Can you work these out from the model? Positions are in its coordinate system, mm. A direction names the side the tool comes from. Give positions to 0.01 mm unless a question says otherwise; leave off trailing zeros. Loops run counter-clockwise (first coordinate to the right, second up) from the corner with the lowest first, then second, coordinate; pieces in that order, holes last. Notation, with made-up numbers: M -22.5,-15.75 L 8.5,-15.75 A14 ccw 8.5,3.25 Z; hole C 46,-10.75 d3. An arc over 180 degrees is marked long. Put each result on its own line as item: value. Start each with the question number.
1) Imagine slicing it at A-A (x = 6). Write out the boundary of the cut face in (y, z), then the cut area to 3 significant figures.
2) Imagine slicing it at B-B (y = -6). State how many separate pieces and enclosed holes the cut face has, then the cut area to 3 significant figures.
3) For faces 1 (the cylindrical face through (15.32, -11.43, 4.4)), 2 (the cylindrical face through (1.5, -1.43, 2.49)), 3 (the cylindrical face through (15.32, -11.43, 0.6)), 4 (the cylindrical face through (72.18, -15.99, 4.43)), 5 (the cylindrical face through (1.43, -10.5, 2.49)), which set-ups out of +Z, -Z, +X, -X, +Y, -Y let a thin tool reach every point of the face, with its end or its side?
4) Please list where these lines run through material, in increasing order: line 1 along Y through (x, z) = (14, 1.85); line 2 along Y through (x, z) = (22.5, 4.65); line 3 along Y through (x, z) = (10, 0.9). Write a range as from..to.
5) For P1, Ø1, axis at x = 60.5, z = 3, coming from the +Y side; P2, Ø4.5, axis at x = 22, y = -6, coming from the +Z side; P3, Ø5, axis at x = 6, y = -6, coming from the -Z side, each with a flat end and sliding along its axis, tell me the tip position at first contact or that it passes through.
6) If we mould it in two halves opening along X, with no side actions, what happens to faces 6 (the cylindrical face through (81.685, -21.377, 4.43)), 7 (the cylindrical face through (0.57, -5.99, 0.6)), 8 (the cylindrical face through (12.4, -7.2, 2.5))? For each: +X half, -X half, draft (parallel to the pull), parting line (faces both ways), or undercut.
from build123d import *

# Parameters (mm, degrees)
F0_W         = 25
F0_H         = 12
F0_W_2       = 15
F1_DEPTH     = 5
F2_R         = 2
F3_DEPTH     = 5.001
F4_R         = 2
F5_T1_DEPTH  = 5
F5_T4_ANGLE  = 90
F5_T6_ANGLE  = 90
F5_T8_ANGLE  = 90
F5_T10_ANGLE = 90
F5_T12_ANGLE = 90
F5_T14_ANGLE = 90
F5_T16_ANGLE = 90
F5_T18_ANGLE = 90
F6_SIZE      = 1


# Not quite as in the source:
# - a fillet or chamfer that OpenCascade refuses, or shapes differently, is made with other operations: its cross-section is extruded or revolved along the edge and cut away or added


with BuildPart() as f1:
    # F0 (on Top) → F1 (new body)
    with BuildSketch(Plane.XY):
        with Locations((12.5, -6)):
            Rectangle(F0_W, F0_H)
        Polygon((67.2861679354, -15.3909064497), (25, 0), (25, -12), (67.2861679354, -27.3909064497), align=None)
        with Locations((74.7861679354, -21.3909064497)):
            Rectangle(F0_W_2, F0_H)
    extrude(amount=F1_DEPTH)

    # F2 (on face) → F3 (cut, through all)
    with BuildSketch(Plane.XY.offset(5)):
        with Locations((6, -6)):
            Circle(F2_R)
        with Locations((76.2861679354, -21.3909064497)):
            Circle(F2_R)
        with Locations((14, -6)):
            Circle(F2_R)
        with Locations((22, -6)):
            Circle(F2_R)
        with Locations((68.2861679354, -21.3909064497)):
            Circle(F2_R)
    extrude(amount=-F3_DEPTH, mode=Mode.SUBTRACT)

    # F4
    f4_edges = [f1.edges().sort_by_distance(p)[0] for p in [
        (46.143084, -7.695453, 5),
        (74.786168, -15.390906, 5),
        (82.286168, -21.390906, 5),
        (74.786168, -27.390906, 5),
        (46.143084, -19.695453, 5),
        (12.5, -12, 5),
        (0, -6, 5),
        (12.5, 0, 5),
        (12.5, -12, 0),
        (0, -6, 0),
        (12.5, 0, 0),
        (46.143084, -7.695453, 0),
        (46.143084, -19.695453, 0),
        (74.786168, -27.390906, 0),
        (74.786168, -15.390906, 0),
        (82.286168, -21.390906, 0),
    ]]
    fillet(f4_edges, radius=F4_R)

    # F5: fillet of radius 5 on 4 edges, made by hand

    # F5_s2 → F5_t1 (cut)
    with BuildSketch(Plane.XY):
        with BuildLine():
            ThreePointArc((77.2861679354, -15.3909064497), (80.8217018413, -16.8553725437), (82.2861679354, -20.3909064497))
            Line((82.2861679354, -20.3909064497), (82.2861679354, -15.3909064497))
            Line((82.2861679354, -15.3909064497), (77.2861679354, -15.3909064497))
        make_face()
        with BuildLine():
            ThreePointArc((82.2861679354, -22.3909064497), (80.8217018413, -25.9264403556), (77.2861679354, -27.3909064497))
            Line((77.2861679354, -27.3909064497), (82.2861679354, -27.3909064497))
            Line((82.2861679354, -27.3909064497), (82.2861679354, -22.3909064497))
        make_face()
        with BuildLine():
            ThreePointArc((0, -7), (1.4644660941, -10.5355339059), (5, -12))
            Line((5, -12), (0, -12))
            Line((0, -12), (0, -7))
        make_face()
        with BuildLine():
            ThreePointArc((5, 0), (1.4644660941, -1.4644660941), (0, -5))
            Line((0, -5), (0, 0))
            Line((0, 0), (5, 0))
        make_face()
    extrude(amount=F5_T1_DEPTH, mode=Mode.SUBTRACT)

    # F5_s3 → F5_t4 (revolve, cut)
    with BuildSketch(Plane.XZ.offset(5)):
        with BuildLine():
            ThreePointArc((2, 0), (0.5857864376, 0.5857864376), (0, 2))
            Line((0, 2), (0, 0))
            Line((0, 0), (2, 0))
        make_face()
    revolve(axis=Axis((5, -5, 0), (0, 0, -1)), revolution_arc=F5_T4_ANGLE, mode=Mode.SUBTRACT)

    # F5_s5 → F5_t6 (revolve, cut)
    with BuildSketch(Plane.YZ.offset(5)):
        with BuildLine():
            ThreePointArc((-10, 0), (-11.4142135624, 0.5857864376), (-12, 2))
            Line((-12, 2), (-12, 0))
            Line((-12, 0), (-10, 0))
        make_face()
    revolve(axis=Axis((5, -7, 0), (0, 0, -1)), revolution_arc=F5_T6_ANGLE, mode=Mode.SUBTRACT)

    # F5_s7 → F5_t8 (revolve, cut)
    with BuildSketch(Plane.XZ.offset(22.3909064497)):
        with BuildLine():
            ThreePointArc((80.2861679354, 0), (81.7003814977, 0.5857864376), (82.2861679354, 2))
            Line((82.2861679354, 2), (82.2861679354, 0))
            Line((82.2861679354, 0), (80.2861679354, 0))
        make_face()
    revolve(axis=Axis((77.2861679354, -22.3909064497, 0), (0, 0, -1)), revolution_arc=F5_T8_ANGLE, mode=Mode.SUBTRACT)

    # F5_s9 → F5_t10 (revolve, cut)
    with BuildSketch(Plane.YZ.offset(77.2861679354)):
        with BuildLine():
            ThreePointArc((-17.3909064497, 0), (-15.9766928873, 0.5857864376), (-15.3909064497, 2))
            Line((-15.3909064497, 2), (-15.3909064497, 0))
            Line((-15.3909064497, 0), (-17.3909064497, 0))
        make_face()
    revolve(axis=Axis((77.2861679354, -20.3909064497, 0), (0, 0, -1)), revolution_arc=F5_T10_ANGLE, mode=Mode.SUBTRACT)

    # F5_s11 → F5_t12 (revolve, cut)
    with BuildSketch(Plane.XZ.offset(20.3909064497)):
        with BuildLine():
            ThreePointArc((80.2861679354, 5), (81.7003814977, 4.4142135624), (82.2861679354, 3))
            Line((82.2861679354, 3), (82.2861679354, 5))
            Line((82.2861679354, 5), (80.2861679354, 5))
        make_face()
    revolve(axis=Axis((77.2861679354, -20.3909064497, 5), (0, 0, 1)), revolution_arc=F5_T12_ANGLE, mode=Mode.SUBTRACT)

    # F5_s13 → F5_t14 (revolve, cut)
    with BuildSketch(Plane.YZ.offset(77.2861679354)):
        with BuildLine():
            ThreePointArc((-25.3909064497, 5), (-26.805120012, 4.4142135624), (-27.3909064497, 3))
            Line((-27.3909064497, 3), (-27.3909064497, 5))
            Line((-27.3909064497, 5), (-25.3909064497, 5))
        make_face()
    revolve(axis=Axis((77.2861679354, -22.3909064497, 5), (0, 0, 1)), revolution_arc=F5_T14_ANGLE, mode=Mode.SUBTRACT)

    # F5_s15 → F5_t16 (revolve, cut)
    with BuildSketch(Plane.XZ.offset(7)):
        with BuildLine():
            ThreePointArc((2, 5), (0.5857864376, 4.4142135624), (0, 3))
            Line((0, 3), (0, 5))
            Line((0, 5), (2, 5))
        make_face()
    revolve(axis=Axis((5, -7, 5), (0, 0, 1)), revolution_arc=F5_T16_ANGLE, mode=Mode.SUBTRACT)

    # F5_s17 → F5_t18 (revolve, cut)
    with BuildSketch(Plane.YZ.offset(5)):
        with BuildLine():
            ThreePointArc((-2, 5), (-0.5857864376, 4.4142135624), (0, 3))
            Line((0, 3), (0, 5))
            Line((0, 5), (-2, 5))
        make_face()
    revolve(axis=Axis((5, -5, 5), (0, 0, 1)), revolution_arc=F5_T18_ANGLE, mode=Mode.SUBTRACT)

    # F6
    f6_edges = [f1.edges().sort_by_distance(p)[0] for p in [
        (20, -6, 5),
        (24, -6, 2.5),
        (20, -6, 0),
        (12, -6, 5),
        (16, -6, 2.5),
        (12, -6, 0),
        (4, -6, 5),
        (8, -6, 2.5),
        (4, -6, 0),
        (66.286168, -21.390906, 5),
        (70.286168, -21.390906, 2.5),
        (66.286168, -21.390906, 0),
        (74.286168, -21.390906, 5),
        (78.286168, -21.390906, 2.5),
        (74.286168, -21.390906, 0),
    ]]
    chamfer(f6_edges, length=F6_SIZE)


solid = f1.part
Recorded:
1. outline: M -12,2 A2 ccw -10,0 L -9,0 L -8,1 L -8,4 L -9,5 L -10,5 A2 ccw -12,3 Z; M -4,1 L -3,0 L -2,0 A2 ccw 0,2 L 0,3 A2 ccw -2,5 L -3,5 L -4,4 Z
1. area: 34.6 mm²
2. separate pieces: 4
2. enclosed holes: 0
2. area: 135 mm²
3. face 1: +Z, -X, -Y
3. face 2: +Z, -Z, -X, +Y
3. face 3: -Z, -X, -Y
3. face 4: +Z, +X, +Y
3. face 5: +Z, -Z, -X, -Y
4. line 1: -11.99..-8, -4..-0.01
4. line 2: -11.13..-8.6, -3.4..-0.87
4. line 3: -11.67..-0.33
5. P1: y = -12.74
5. P2: z = 4.25
5. P3: z = 0.5
6. face 6: +X half
6. face 7: -X half
6. face 8: undercut
